Part model, mm, in its own coordinate system. A direction names the side the tool comes from. Give positions to 0.01 mm unless a question says otherwise; leave off trailing zeros. Write each loop counter-clockwise with the first axis right and the second up, starting at its lowest first coordinate (ties: lowest second). Pieces come first, ordered by that corner, then holes. Notation, with made-up numbers: (72, 44) - (76, 44) arc R21 cw to (76, 48) - close; hole circle Ø10 at (88, 40). An arc over 180 degrees is marked (long way). Answer as a JSON object with one key per item and string values. Group by question number.
```python
from build123d import *

# Parameters (mm, degrees)
ESQUISSE1_R                  = 35
ESQUISSE1_R_2                = 10
BOSS_EXTRU_1_DEPTH           = 20
ESQUISSE2_R                  = 22.5
ENL_V_MAT_EXTRU_1_DEPTH      = 15
ESQUISSE3_R                  = 4
ENL_V_MAT_EXTRU_2_DEPTH      = 56.452682532
R_P_TITION_CIRCULAIRE1_COUNT = 5


with BuildPart() as part:
    # Esquisse1 → Boss.-Extru.1 (new, symmetric)
    with BuildSketch(Plane.XY):
        Circle(ESQUISSE1_R)
        Circle(ESQUISSE1_R_2, mode=Mode.SUBTRACT)
    extrude(amount=BOSS_EXTRU_1_DEPTH, both=True)

    # Esquisse2 → Enlèv. mat.-Extru.1 (cut)
    with BuildSketch(Plane.XY.offset(20)):
        Circle(ESQUISSE2_R)
    enl_v_mat_extru_1 = extrude(amount=-ENL_V_MAT_EXTRU_1_DEPTH, mode=Mode.SUBTRACT)

    # Symétrie1: Enlèv. mat.-Extru.1 across plane
    add(enl_v_mat_extru_1.mirror(Plane.XY), mode=Mode.SUBTRACT)

    # Esquisse3 → Enlèv. mat.-Extru.2 (cut, through all)
    with BuildSketch(Plane.XY.offset(5)):
        with Locations((0, 16.5)):
            Circle(ESQUISSE3_R)
    enl_v_mat_extru_2 = extrude(amount=-ENL_V_MAT_EXTRU_2_DEPTH, mode=Mode.SUBTRACT)

    # Répétition circulaire1: Enlèv. mat.-Extru.2 ×5 about axis
    r_p_tition_circulaire1_axis = Axis((0, 0, 0), (0, 0, 1))
    for i in range(1, R_P_TITION_CIRCULAIRE1_COUNT):
        add(enl_v_mat_extru_2.rotate(r_p_tition_circulaire1_axis, i * 360 / R_P_TITION_CIRCULAIRE1_COUNT), mode=Mode.SUBTRACT)

    # Esquisse4 → Enlèvement de matière-Révolution1 (revolve, cut)
    with BuildSketch(Plane(origin=(0, 0, 0), x_dir=(1, 0, 0), z_dir=(0, 1, 0)), mode=Mode.PRIVATE) as enl_vement_de_mati_re_r_volution1_sk:
        Polygon((35, 17), (29, 13.535898385), (29, -13.535898385), (35, -17), align=None)
    revolve(enl_vement_de_mati_re_r_volution1_sk.sketch.rotate(Axis((0, 0, -37.926889672), (0, 0, 1)), 180), axis=Axis((0, 0, -37.926889672), (0, 0, 1)), mode=Mode.SUBTRACT)


solid = part.part
```
1) Band-saw the part on B-B (x = 0). List the corners of the cut face in (y, z).
2) Probe line 1 (Y direction, x = 0, z = 11); line 2 (Z direction, x = -22, y = -3.5); line 3 (Z direction, x = -12, y = -29). List the from-to ranges inside material, lowest first.
3) Which spindle directions (+Z, -Z, +X, -X, +Y, -Y) get a long thin tool onto all of the face, cutting with end or side? Do faces 4 (the cylindrical face through (-2.17, -9.76, -0.07)), 5 (the cylindrical face through (10.382, -19.961, -12.605)), 6 (the flat face through (0, -23, -20)), 7 (the cylindrical face through (10.382, -19.961, 12.605)), 8 (the conical face through (6.368, 28.677, 13.753)). Say none if no direction does.
4) Band-saw the part on D-D (z = 3.5). List the corners of the cut face in (x, y), plus the area to 3 significant figures.
5) Drop flat-ended pins along their axis: P1, Ø1.5, axis at x = 26, z = -3.5, coming from the -Y side; P2, Ø10.5, axis at x = -15.69, y = 5.1, coming from the -Z side; P3, Ø6.5, axis at x = -9.7, y = -13.35, coming from the -Z side; P4, Ø10, axis at x = -4, y = 14, coming from the +Z side. Give the stop position or say it passes through.
6) Band-saw the part on C-C (z = -11.5). List the corners of the cut face in (x, y).
7) Mould opens along X. For faces 1 (the cylindrical face through (-28, -21, 19)), 2 (the flat face through (0, -23, 20)), 3 (the flat face through (-10.3, 0.3, 5)) say: pulls with the +X half, pulls with the -X half, needs draft (parallel to the pull), parting line crosses it, or undercut.
8) Band-saw the part on A-A (y = 0). List the corners of the cut face in (x, z).
Verdict:
{
 "1": {"outline": "(-35, -20) - (-22.5, -20) - (-22.5, -5) - (-10, -5) - (-10, 5) - (-22.5, 5) - (-22.5, 20) - (-35, 20) - (-35, 17) - (-29, 13.54) - (-29, -13.54) - (-35, -17) - close; (10, -5) - (12.5, -5) - (12.5, 5) - (10, 5) - close; (20.5, -5) - (22.5, -5) - (22.5, -20) - (35, -20) - (35, -17) - (29, -13.54) - (29, 13.54) - (35, 17) - (35, 20) - (22.5, 20) - (22.5, 5) - (20.5, 5) - close"},
 "2": {"line 1": "-29 to -22.5, 22.5 to 29", "line 2": "-5 to 5", "line 3": "-20 to -14.91, 14.91 to 20"},
 "3": {"face 4": "+Z, -Z", "face 5": "-Z", "face 6": "-Z, +X, -X, +Y, -Y", "face 7": "+Z", "face 8": "none"},
 "4": {"outline": "circle Ø58 at (0, 0); hole circle Ø8 at (-15.69, 5.1); hole circle Ø8 at (-9.7, -13.35); hole circle Ø20 at (0, 0); hole circle Ø8 at (0, 16.5); hole circle Ø8 at (9.7, -13.35); hole circle Ø8 at (15.69, 5.1)", "area": "2,080 mm2"},
 "5": {"P1": "y = -14.26", "P2": "z = -5", "P3": "through", "P4": "z = 5"},
 "6": {"outline": "circle Ø58 at (0, 0); hole circle Ø45 at (0, 0)"},
 "7": {"face 1": "parting line crosses it", "face 2": "needs draft", "face 3": "undercut"},
 "8": {"outline": "(-35, -20) - (-22.5, -20) - (-22.5, -5) - (-10, -5) - (-10, 5) - (-22.5, 5) - (-22.5, 20) - (-35, 20) - (-35, 17) - (-29, 13.54) - (-29, -13.54) - (-35, -17) - close; (10, -5) - (22.5, -5) - (22.5, -20) - (35, -20) - (35, -17) - (29, -13.54) - (29, 13.54) - (35, 17) - (35, 20) - (22.5, 20) - (22.5, 5) - (10, 5) - close"}
}
